from build123d import *

# Parameters (mm, degrees)
SKETCH_2_R          = 1.6
CUT_EXTRUDE_1_DEPTH = 42


with BuildPart() as part:
    # 草图1 → 旋转1 (revolve)
    with BuildSketch(Plane.XY, mode=Mode.PRIVATE) as revolve_1_sk:
        Polygon((0, 14.96953125), (10, 14.96953125), (10, 13.96953125), (7.5, 13.96953125), (7.5, -16.23046875), (0, -16.23046875), align=None)
    revolve(revolve_1_sk.sketch.rotate(Axis((0, -16.23046875, 0), (0, 1, 0)), 90), axis=Axis((0, -16.23046875, 0), (0, 1, 0)))

    # 草图2 → 切除-拉伸1 (cut)
    with BuildSketch(Plane.XZ.offset(16.23046875)):
        with Locations(Location((0, 4, 0), (0, 0, 270))):
            Circle(SKETCH_2_R)
        with Locations(Location((0, -4, 0), (0, 0, 270))):
            Circle(SKETCH_2_R)
    extrude(amount=-CUT_EXTRUDE_1_DEPTH, mode=Mode.SUBTRACT)


solid = part.part
Geometry check sheet. Reference: the model listing, model coordinates, mm. A direction names the side the tool comes from. Round coordinates to 2 decimals unless told otherwise and drop trailing zeros. Loops run counter-clockwise (first coordinate to the right, second up) from the corner with the lowest first, then second, coordinate; pieces in that order, holes last. Notation, with made-up numbers: (4, 15.25) -> (62, 15.25) arc R30 cw to (62, 40.25) -> close; hole circle Ø2 at (39.25, 74.25). An arc over 180 degrees is marked (long way). Answer as a JSON object with one key per item and string values. Group by question number.
Item 1: Cross-section at D-D, the plane x = 6. Record the cut outline in (y, z).
Item 2: Depth check by flat-ended pin: pin 1 Ø12 at (x, y) = (-8, -11) entering from +Z; pin 2 Ø3 at (x, y) = (2.5, -12.5) entering from +Z; pin 3 Ø4 at (x, y) = (5.5, 11.5) entering from +Z. Enter the tip coordinate at first touch or a pass-through.
Item 3: Set-up check for faces 1 (the face through (-0.61, -0.85, -5.48)), 2 (the face through (-7, 13.97, -4)): record each of +Z, -Z, +X, -X, +Y, -Y from which the full face is reachable in a straight line by a thin tool's end or side.
Item 4: Release check for a two-part mould opening along Z. For faces 3 (the face through (-0.97, -0.85, 5.27)), 4 (the face through (0, -16.23, 0)), 5 (the face through (-0.44, 14.46, 9.99)) record: pulls with the +Z half, pulls with the -Z half, needs draft (parallel to the pull), parting line crosses it, or undercut.
Item 5: Cross-section at B-B, the plane z = 4. Record the cut outline in (x, y).
Item 6: Cross-section at C-C, the plane y = -3. Record the cut outline in (x, z), plus the area to 3 significant figures.
Item 7: Thickness scan on line 1 along X through (y, z) = (9, -4); line 2 along Y through (x, z) = (-5, -8); line 3 along X through (y, z) = (1, -0.25). Record the ranges inside material, lowest first.
Item 8: Cross-section at A-A, the plane x = 0. Record the cut outline in (y, z).
Determined:
{
 "1": {"outline": "(-16.23, -4.5) -> (13.97, -4.5) -> (13.97, -8) -> (14.97, -8) -> (14.97, 8) -> (13.97, 8) -> (13.97, 4.5) -> (-16.23, 4.5) -> close"},
 "2": {"pin 1": "stops at z = 7.23", "pin 2": "stops at z = 7.43", "pin 3": "stops at z = 6.63"},
 "3": {"face 1": "+Y, -Y", "face 2": "-Y"},
 "4": {"face 3": "undercut", "face 4": "needs draft", "face 5": "parting line crosses it"},
 "5": {"outline": "(-9.17, 13.97) -> (-6.34, 13.97) -> (-6.34, -16.23) -> (-1.6, -16.23) -> (-1.6, 14.97) -> (-9.17, 14.97) -> close; (1.6, -16.23) -> (6.34, -16.23) -> (6.34, 13.97) -> (9.17, 13.97) -> (9.17, 14.97) -> (1.6, 14.97) -> close"},
 "6": {"outline": "circle Ø15 at (0, 0); hole circle Ø3.2 at (0, -4); hole circle Ø3.2 at (0, 4)", "area": "161 mm²"},
 "7": {"line 1": "x = -6.34 to -1.6, 1.6 to 6.34", "line 2": "y = 13.97 to 14.97", "line 3": "x = -7.5 to 7.5"},
 "8": {"outline": "(-16.23, -7.5) -> (13.97, -7.5) -> (13.97, -10) -> (14.97, -10) -> (14.97, -5.6) -> (-16.23, -5.6) -> close; (-16.23, -2.4) -> (14.97, -2.4) -> (14.97, 2.4) -> (-16.23, 2.4) -> close; (-16.23, 5.6) -> (14.97, 5.6) -> (14.97, 10) -> (13.97, 10) -> (13.97, 7.5) -> (-16.23, 7.5) -> close"}
}
